Design review of the part built by this model. Coordinates are the model's own, in mm. Face numbers are marked on the shaded views. A direction names the side the tool comes from. Coordinates: 2 decimals unless noted, no trailing zeros. Write each loop counter-clockwise with the first axis right and the second up, starting at its lowest first coordinate (ties: lowest second). Pieces come first, ordered by that corner, then holes. Notation, with made-up numbers: (6, 58.5) - (19, 58.5) arc R28 cw to (19, 90.5) - close; hole circle Ø9 at (14.25, 68). An arc over 180 degrees is marked (long way). One line per item, written item: value.
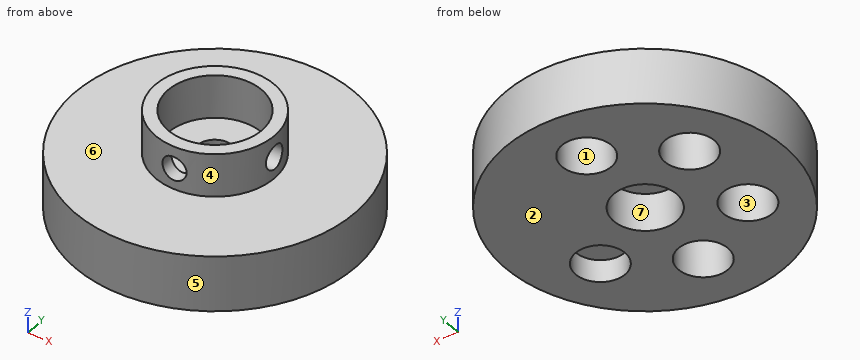
Autodesk Fusion 360 part; units mm, degrees
sketch "Sketch1" plane through (0, 0, 0) normal (0, 0, 1) x (1, 0, 0)
  circle A0 centre (0, 0) radius 20
  circle A1 centre (0, -12) radius 3.55
  circle A2 centre (0, 12) radius 3.55
  circle A3 centre (10.3923, -6) radius 3.55
  circle A4 centre (-10.3923, 6) radius 3.55
  circle A5 centre (-10.3923, -6) radius 3.55
  circle A6 centre (0, 0) radius 2.1
  line L0 (0, 0) -> (0, 12) construction
  line L1 (0, 0) -> (10.3923, -6) construction
  line L2 (0, 0) -> (10.3923, 6) construction
  circle A7 centre (10.3923, 6) radius 3.55
  dimension "d1" = 40
  dimension "d2" = 7.1
  dimension "d3" = 7.1
  dimension "d6" = 7.1
  dimension "d12" = 12
  dimension "d15" = 12
  dimension "d16" = 7.1
  dimension "d17" = 12
  dimension "d19" = 7.1
  dimension "d23" = 12
  dimension "d25" = 4.2
  dimension "d34" = 60
  dimension "d37" = 60
  dimension "d38" = 60
  dimension "d39" = 60
  dimension "d49" = 12
  dimension "d50" = 7.1
  dimension "d51" = 60
  dimension "d52" = 60
  dimension "d85" = 12
sketch "Sketch2" plane through (0, 0, 0) normal (0, 0, 1) x (1, 0, 0)
  circle A0 centre (0, 0) radius 20
  line L0 (0, 0) -> (0, -9) construction
  line L1 (0, 0) -> (0, 9) construction
  line L2 (20, -0.0372) -> (-20, -0.0372) construction
  line L3 (-14, -0.0372) -> (-20, -0.0372) construction
  dimension "d26" = 40
  dimension "d40" = 6
extrude "Extrude1" add sketch "Sketch2" along normal blind 5 and the other way blind 3
sketch "Sketch3" plane through (0, 0, 0) normal (0, 0, 1) x (1, 0, 0)
hole "Hole1" at (-0.003, -0.037, -3) direction (0, 0, 1) diameter 5.029 depth 14 tip angle 180 counterbore diameter 9 counterbore depth 5.4
extrude "Extrude2" cut sketch "Sketch1" along normal blind -3 and the other way blind -0.2 contours A1 | A2 | A3 | A4 | A5
extrude "Extrude4" cut sketch "Sketch1" along normal blind 0.2 and the other way blind 3 contours A7
sketch "Sketch4" plane through (0, 0, 5) normal (0, 0, 1) x (-1, 0, 0)
  circle A0 centre (0.003, 0.037) radius 2.5143
  circle A1 centre (0, 0) radius 20
  circle A2 centre (0, 0) radius 6.5
  circle A3 centre (0, 0) radius 3
  dimension "d57" = 13
  dimension "d58" = 6
sketch "Sketch5" plane through (0, 0, 5) normal (0, 0, 1) x (-1, 0, 0)
  circle A0 centre (0, 0) radius 20
  circle A1 centre (0, 0) radius 8.5
  circle A2 centre (0, 0) radius 6.7
  circle A3 centre (0.003, 0.037) radius 2.5143
  dimension "d61" = 17
  dimension "d62" = 13.4
extrude "Extrude6" add sketch "Sketch5" along normal blind 6.2 contours A1
sketch "Sketch6" plane through (0, 0, 5) normal (0, 0, 1) x (-1, 0, 0)
  circle A0 centre (0, 0) radius 20
  circle A1 centre (0, 0) radius 8.5
  circle A2 centre (0, 0) radius 6.5
  dimension "d65" = 13
sketch "Sketch7" plane through (0, 0, 0) normal (1, 0, 0) x (0, 1, 0)
sketch "Sketch8" plane through (0, 0, 11.2) normal (0, 0, 1) x (-1, 0, 0)
  circle A0 centre (0, 0) radius 6.7
  circle A1 centre (0, 0) radius 8.5
sketch "Sketch9" plane through (0, 0, 11.2) normal (0, 0, 1) x (-1, 0, 0)
  line L0 (0, -8.4831) -> (0, 8.4366) construction
  line L1 (8.5, -0.0044) -> (-8.5, -0.0044) construction
  circle A0 centre (0, 0) radius 8.5 construction
  arc A1 (0, -8.4831) -> (6.3875, -5.608) centre (0.0534, -0.0686) ccw
extrude "Extrude3" cut sketch "Sketch1" along normal blind 3.2 contours A1 | A2 | A3 | A4 | A5 | A7
sketch "Sketch10" plane through (0, 0, 0) normal (1, 0, 0) x (0, 1, 0)
  circle A0 centre (0.01, 9) radius 1.5
  line L0 (0, 1.9) -> (0, 14.3)
  circle A1 centre (0.01, 9) radius 1.25
  dimension "d66" = 3
  dimension "d67" = 0.01
  dimension "d68" = 2.5
sketch "Sketch11" plane through (0, 0, 0) normal (0, 1, 0) x (1, 0, 0)
  line L0 (0, -5) -> (0, -11) construction
  line L1 (0, -5) -> (0, -11) construction
  line L2 (0, -5) -> (0, -8) construction
  circle A0 centre (0, -8) radius 1.25
  circle A1 centre (0, -8) radius 1.7
  dimension "d69" = 3
  dimension "d70" = 2.5
  dimension "d86" = 3.4
extrude "Extrude7" cut sketch "Sketch11" against normal blind 19 contours A0
sketch "Sketch12" plane through (0, 0, 0) normal (1, 0, 0) x (0, 1, 0)
  line L0 (0, 5) -> (0, 11)
  line L1 (0, 11) -> (0, 8)
  circle A0 centre (0, 8) radius 1.25
  circle A1 centre (0, 8) radius 1.7
  dimension "d73" = 3
  dimension "d74" = 2.5
  dimension "d89" = 3.4
extrude "Extrude8" cut sketch "Sketch12" along normal blind 18 contours L0 L1 A0 | L0 L1 A0
extrude "Extrude9" cut sketch "Sketch11" against normal blind 11
extrude "Extrude10" cut sketch "Sketch12" along normal blind 15 contours L0 L1 A0 A1 | L0 L1 A0 A1
extrude "Extrude11" add 3 faces at (9.7613, 6.2168, 3.2) (9.7613, 6.2168, 3.2) (9.7613, 6.2168, 3.2) along direction (0, 0, -1) blind 6.2
extrude "Extrude12" add 3 faces at (9.1513, -4.7203, 3.2) (9.1513, -4.7203, 3.2) (9.1513, -4.7203, 3.2) along direction (0, 0, -1) blind 3
thread "Thread3" [suppressed]
1. Mouldability with a two-part tool opening along X and no side actions: class the marked faces 1, 2, 3 and 4 as released by +X, released by -X, zero draft, split by the parting line, or undercut.
Answer block:
face 1: undercut
face 2: zero draft
face 3: undercut
face 4: split by the parting line
2. For the marked faces 5, 6 and 7, list the 3-axis set-ups (+Z, -Z, +X, -X, +Y, -Y) from which the entire face can be reached by the end or side of a thin tool; tool diameter is ignored.
Answer block:
face 5: +Z, -Z
face 6: +Z
face 7: -Z
3. Wall thickness on line 1 along Y through (x, z) = (0, 1.5); line 2 along X through (y, z) = (-5, -2.25); line 3 along Y through (x, z) = (-1, 2): over which ranges is each line inside the solid? List them lowest first.
Answer block:
line 1: y = -20 to -15.55, -8.45 to -4.54, 4.46 to 8.45, 15.55 to 20
line 2: x = -19.36 to -13.8, -6.99 to 6.99, 13.8 to 19.36
line 3: y = -19.97 to -15.41, -8.59 to -4.43, 4.35 to 8.59, 15.41 to 19.97
4. Consider section A-A, the plane y = 12. Write out the cut boundary in (x, z).
Answer block:
outline: (-16, -3) - (-3.55, -3) - (-3.55, 3.2) - (3.55, 3.2) - (3.55, -3) - (16, -3) - (16, 5) - (-16, 5) - close
5. Consider section D-D, the plane z = -0.75. Write out the cut boundary in (x, y), then the cut area to 3 significant figures.
Answer block:
outline: circle Ø40 at (0, 0); hole circle Ø7.1 at (-10.39, -6); hole circle Ø7.1 at (-10.39, 6); hole circle Ø9 at (0, -0.04); hole circle Ø7.1 at (0, -12); hole circle Ø7.1 at (0, 12); hole circle Ø7.1 at (10.39, -6)
area: 995 mm^2
6. Consider section B-B, the plane z = 7.25. Write out the cut boundary in (x, y).
Answer block:
outline: (-1.53, -8.36) - (-1.53, -6.52) arc R6.7 cw (long way) to (6.52, 1.53) - (8.36, 1.53) arc R8.5 ccw (long way) to start; (1.53, -8.36) arc R8.5 ccw to (8.36, -1.53) - (6.52, -1.53) arc R6.7 cw to (1.53, -6.52) - close
7. Consider section C-C, the plane y = 0. Write out the cut boundary in (x, z), then the cut area to 3 significant figures.
Answer block:
outline: (-20, -3) - (-4.5, -3) - (-4.5, 2.4) - (-2.52, 2.4) - (-2.52, 5) - (-6.7, 5) - (-6.7, 11.2) - (-8.5, 11.2) - (-8.5, 5) - (-20, 5) - close; (2.51, 2.4) - (4.5, 2.4) - (4.5, -3) - (20, -3) - (20, 5) - (8.5, 5) - (8.5, 6.3) - (6.7, 6.3) - (6.7, 5) - (2.51, 5) - close; (6.7, 9.7) - (8.5, 9.7) - (8.5, 11.2) - (6.7, 11.2) - close
area: 275 mm^2
8. Insertion check: pin 1 Ø3.5 at (x, y) = (-10, -6.5) entering from -Z; pin 2 Ø2 at (x, z) = (10, 5) entering from -Y; pin 3 Ø8 at (x, y) = (-0.003, -0.037) entering from -Z. Each pin has a flat end and moves straight along its axis. Give the tip position at first contact, or say it passes through.
Answer block:
pin 1: stops at z = 3.2
pin 2: stops at y = -17.86
pin 3: stops at z = 2.4
